```python
from build123d import *

# Parameters (mm, degrees)
SKETCH2_W           = 203.2
SKETCH2_H           = 101.6
SKETCH2_W_2         = 31.75
SKETCH2_H_2         = 50.8
SKETCH2_W_3         = 31.808931498
BOSS_EXTRUDE1_DEPTH = 6.35
SKETCH3_R           = 3.175
CUT_EXTRUDE1_DEPTH  = 34.544
SKETCH5_W           = 69.874867022
SKETCH5_H           = 25.509122939
CUT_EXTRUDE2_DEPTH  = 34.544
SKETCH6_W           = 25.4
SKETCH6_H           = 12.7
CUT_EXTRUDE3_DEPTH  = 34.544


with BuildPart() as part:
    # Sketch2 → Boss-Extrude1 (new body)
    with BuildSketch(Plane(origin=(0, 0, 0), x_dir=(1, 0, 0), z_dir=(0, 1, 0))):
        with Locations((101.6, 50.8)):
            Rectangle(SKETCH2_W, SKETCH2_H)
        with Locations((28.575, 50.8)):
            Rectangle(SKETCH2_W_2, SKETCH2_H_2, mode=Mode.SUBTRACT)
        with Locations((173.511909894, 50.8)):
            Rectangle(SKETCH2_W_3, SKETCH2_H_2, mode=Mode.SUBTRACT)
    extrude(amount=BOSS_EXTRUDE1_DEPTH)

    # Sketch3 → Cut-Extrude1 (cut)
    with BuildSketch(Plane(origin=(0, 6.35, 0), x_dir=(1, 0, 0), z_dir=(0, 1, 0))):
        with Locations(Location((69.85, 76.2, 0), (0, 0, 270))):
            Circle(SKETCH3_R)
        with Locations(Location((133.35, 76.2, 0), (0, 0, 270))):
            Circle(SKETCH3_R)
    extrude(amount=-CUT_EXTRUDE1_DEPTH, mode=Mode.SUBTRACT)

    # Sketch5 → Cut-Extrude2 (cut)
    with BuildSketch(Plane(origin=(0, 6.35, 0), x_dir=(1, 0, 0), z_dir=(0, 1, 0))):
        with Locations((101.604794403, 50.641324615)):
            Rectangle(SKETCH5_W, SKETCH5_H)
    extrude(amount=-CUT_EXTRUDE2_DEPTH, mode=Mode.SUBTRACT)

    # Sketch6 → Cut-Extrude3 (cut)
    with BuildSketch(Plane(origin=(0, 6.35, 0), x_dir=(1, 0, 0), z_dir=(0, 1, 0))):
        with Locations((101.6, 19.05)):
            Rectangle(SKETCH6_W, SKETCH6_H)
    extrude(amount=-CUT_EXTRUDE3_DEPTH, mode=Mode.SUBTRACT)


solid = part.part
```
The listing builds one solid part. Answer for the finished solid, in the listing's coordinates (mm). A direction names the side the tool comes from. Round coordinates to 2 decimals unless told otherwise and drop trailing zeros. Write each loop counter-clockwise with the first axis right and the second up, starting at its lowest first coordinate (ties: lowest second). Pieces come first, ordered by that corner, then holes. Notation, with made-up numbers: (69.5, 36.5) -> (74.5, 36.5) arc R34 ccw to (74.5, 72.5) -> close; hole circle Ø5 at (52, -35.5). An arc over 180 degrees is marked (long way). Answer as a JSON object with one key per item and string values. Group by question number.
Q1. Section D-D (y = 3) is taken. Write down the section's boundary in (x, z) (3 decimals), plus the area to 3 significant figures.
Q2. Which of the six approach directions +Z, -Z, +X, -X, +Y, -Y give full straight-line access (tool end or side, diameter ignored) to faces 4 (the face through (28, 3, -76.2)), 5 (the face through (100, 3, -101.6))?
Q3. Section B-B (z = -40) is taken. Write down the section's boundary in (x, y).
Q4. Section A-A (x = 95.5) is taken. Write down the section's boundary in (y, z), plus the area to 3 significant figures.
Q5. Determine the mould class of faces 1 (the face through (203.2, 3, -50)), 2 (the face through (44.45, 3, -50)), 3 (the face through (100, 6.35, -74)) for opening direction X: pulls with the +X half, pulls with the -X half, needs draft (parallel to the pull), parting line crosses it, or undercut.
Q6. Section C-C (x = 184) is taken. Write down the section's boundary in (y, z).
Q7. This flat-tipped pin is pushed along its axis until it touches: pin 1 Ø6 at (x, z) = (30.5, -70.5) entering from -Y. Where does it stop, or does it pass through?
Q8. Straight lines are drawn through the part: line 1 along Z through (x, y) = (133.35, 2.75) (3 decimals); line 2 along X through (y, z) = (4, -36); line 3 along X through (y, z) = (4.25, -50.5). For each, find the intervals that lie inside material, in ascending order.
Check values:
{
 "1": {"outline": "(0, -101.6) -> (203.2, -101.6) -> (203.2, 0) -> (0, 0) -> close; hole (12.7, -76.2) -> (44.45, -76.2) -> (44.45, -25.4) -> (12.7, -25.4) -> close; hole (66.667, -63.396) -> (136.542, -63.396) -> (136.542, -37.887) -> (66.667, -37.887) -> close; hole circle Ø6.35 at (69.85, -76.2); hole (88.9, -25.4) -> (114.3, -25.4) -> (114.3, -12.7) -> (88.9, -12.7) -> close; hole circle Ø6.35 at (133.35, -76.2); hole (157.607, -76.2) -> (189.416, -76.2) -> (189.416, -25.4) -> (157.607, -25.4) -> close", "area": "15,200 mm^2"},
 "2": {"face 4": "+Y, -Y", "face 5": "-Z, +X, -X, +Y, -Y"},
 "3": {"outline": "(0, 0) -> (12.7, 0) -> (12.7, 6.35) -> (0, 6.35) -> close; (44.45, 0) -> (66.67, 0) -> (66.67, 6.35) -> (44.45, 6.35) -> close; (136.54, 0) -> (157.61, 0) -> (157.61, 6.35) -> (136.54, 6.35) -> close; (189.42, 0) -> (203.2, 0) -> (203.2, 6.35) -> (189.42, 6.35) -> close"},
 "4": {"outline": "(0, -101.6) -> (6.35, -101.6) -> (6.35, -63.4) -> (0, -63.4) -> close; (0, -37.89) -> (6.35, -37.89) -> (6.35, -25.4) -> (0, -25.4) -> close; (0, -12.7) -> (6.35, -12.7) -> (6.35, 0) -> (0, 0) -> close", "area": "403 mm^2"},
 "5": {"face 1": "pulls with the +X half", "face 2": "undercut", "face 3": "needs draft"},
 "6": {"outline": "(0, -101.6) -> (6.35, -101.6) -> (6.35, -76.2) -> (0, -76.2) -> close; (0, -25.4) -> (6.35, -25.4) -> (6.35, 0) -> (0, 0) -> close"},
 "7": {"pin 1": "through"},
 "8": {"line 1": "-101.6 to -79.375, -73.025 to -63.396, -37.887 to 0", "line 2": "0 to 12.7, 44.45 to 157.61, 189.42 to 203.2", "line 3": "0 to 12.7, 44.45 to 66.67, 136.54 to 157.61, 189.42 to 203.2"}
}
